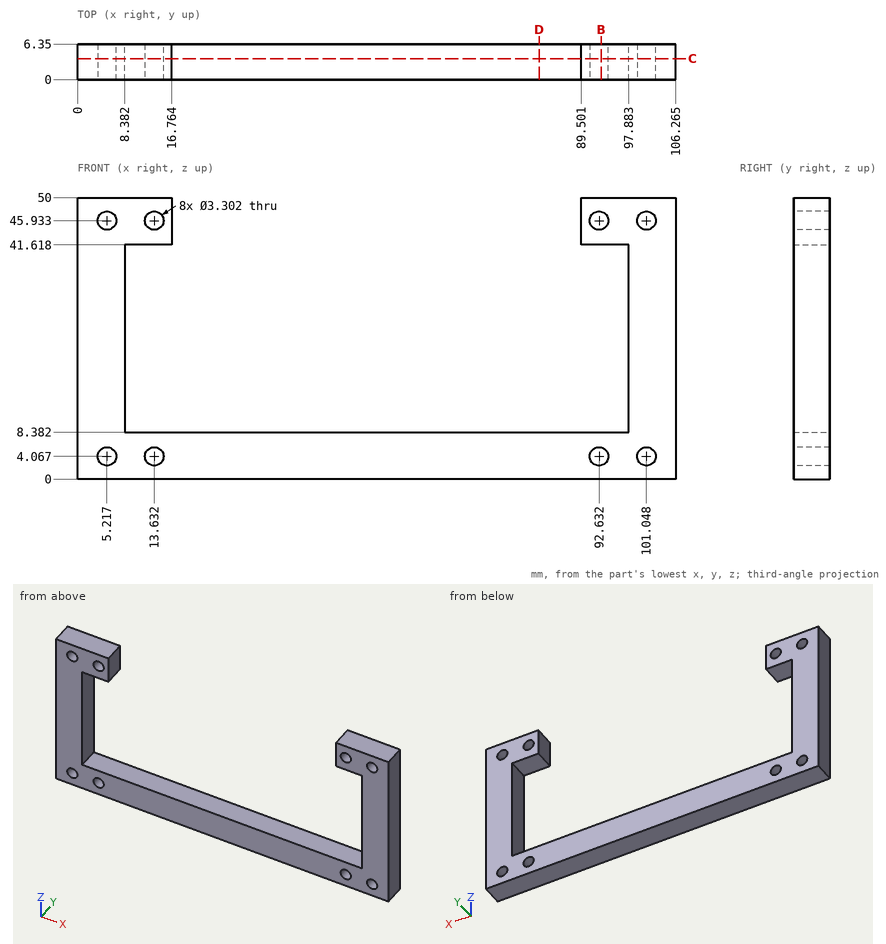
Could you check a few things on this drawing? It's one solid part, dimensions in mm from its lowest x, y, z. Give positions to 0.01 mm unless a question says otherwise; leave off trailing zeros. Order: outer loops, then holes, each group sorted by start corner. A loop starts at its lowest first (then second) coordinate and runs counter-clockwise, first axis right, second up. Notation, with made-up numbers: (45.5, -20) - (57.5, -20) arc R16 cw to (57.5, -14) - close; hole circle Ø4 at (67, -36.75). An arc over 180 degrees is marked (long way). One line per item, written item: value. Start each with the question number.
1. For P1, Ø3, axis at x = 71, y = 3, coming from the +Z side, with a flat end and sliding along its axis, tell me the tip position at first contact or that it passes through.
2. Imagine slicing it at B-B on x = 93. List the corners of the cut face in (y, z) for me.
3. Imagine slicing it at C-C on y = 3.75. Give the number of separate pieces and of enclosed holes in the cut face, plus the area to 3 significant figures.
4. If I drill on probe 1 along X at (y, z) = (4.25, 46) (1 decimal); probe 2 along X at (y, z) = (0.5, 22.5) (1 decimal); probe 3 along X at (y, z) = (1, 43.5) (1 decimal), over which ranges is the centre line in solid material (lowest first)?
5. Imagine slicing it at D-D on x = 82. List the corners of the cut face in (y, z) for me, plus the area to 3 significant figures.
Values:
1. P1: z = 8.38
2. outline: (0, 0) - (6.35, 0) - (6.35, 2.46) - (0, 2.46) - close; (0, 5.68) - (6.35, 5.68) - (6.35, 8.38) - (0, 8.38) - close; (0, 41.62) - (6.35, 41.62) - (6.35, 44.32) - (0, 44.32) - close; (0, 47.54) - (6.35, 47.54) - (6.35, 50) - (0, 50) - close
3. separate pieces: 1
3. enclosed holes: 8
3. area: 1,660 mm²
4. probe 1: 0 to 3.6, 6.9 to 12, 15.3 to 16.8, 89.5 to 91, 94.3 to 99.4, 102.7 to 106.3
4. probe 2: 0 to 8.4, 97.9 to 106.3
4. probe 3: 0 to 16.8, 89.5 to 106.3
5. outline: (0, 0) - (6.35, 0) - (6.35, 8.38) - (0, 8.38) - close
5. area: 53.2 mm²
